Autodesk Inventor part; units mm, degrees
ref_plane "YZ Plane" through (0, 0, 0) normal (1, 0, 0) x (0, 1, 0)
ref_plane "XZ Plane" through (0, 0, 0) normal (0, 1, 0) x (-1, 0, 0)
ref_plane "XY Plane" through (0, 0, 0) normal (0, 0, 1) x (1, 0, 0)
sketch "スケッチ1" plane through (0, 0, 0) normal (0, 0, 1) x (1, 0, 0)
  line L0 (-50, 0) -> (50, 0) construction
  circle A0 centre (-50, 0) radius 4.05
  circle A1 centre (50, 0) radius 4.05
  line L1 (-50, 8.5) -> (43, 8.5)
  line L2 (-50, -8.5) -> (43, -8.5)
  arc A2 (-50, 8.5) -> (-50, -8.5) centre (-50, 0) ccw
  line L3 (43, -8.5) -> (50.119, -8.3992)
  line L4 (43, 8.5) -> (50.119, 8.3992)
  arc A3 (50.119, -8.3992) -> (50.119, 8.3992) centre (50, 0) ccw
  line L5 (-29, -7.5) -> (0, -7.5) construction
  line L6 (0, -7.5) -> (0, -2.5) construction
  line L7 (0, -2.5) -> (-29, -2.5) construction
  line L8 (-29, -2.5) -> (-29, -7.5) construction
  line L9 (-29, -5) -> (0, -5) construction
  circle A4 centre (-26.5, -5) radius 1.55
  line L10 (-14.5, -5) -> (-14.5, -2.5) construction
  line L11 (52.3191, 13) -> (22.3191, 13)
  line L12 (22.3191, 13) -> (12.3191, 8.5)
  line L13 (52.3191, 13) -> (57.3191, 4.122)
  circle A5 centre (-2.5, -5) radius 1.55
  point P0 (0, 0)
  point P1 (0, 0)
  point P2 (54.8534, 8.5)
  dimension "d0" = 100
  dimension "d1" = 8.1
  dimension "d2" = 8.5
  dimension "d8" = 8.1
  dimension "d9" = 7
  dimension "d10" = 8.4
  dimension "d12" = 5
  dimension "d13" = 29
  dimension "d15" = 2.5
  dimension "d17" = 13
  dimension "d19" = 10
  dimension "d20" = 30
  dimension "d25" = 50
  dimension "d26" = 5
  dimension "d45" = 1
  dimension "d46" = 3.1
extrude "押し出し1" add sketch "スケッチ1" along normal blind 2 contours L1 L4 A3 L3 L2 A2
fillet "フィレット1" radius 2 1 edges at (43, 8.5, 1)
sketch "スケッチ2" plane through (0, 0, 0) normal (0, 0, -1) x (-1, 0, 0)
  circle A0 centre (-16.6795, 17.7128) radius 11.35 construction
  circle A1 centre (-16.6795, 17.7128) radius 11.55
  line L0 (-16.6795, 6.1628) -> (58.7547, 6.1628)
  line L1 (-16.6795, 17.7128) -> (-34, 27.7128) construction
  circle A2 centre (-50, 0) radius 4.05
  line L2 (-50, 0) -> (-34, 27.7128) construction
  line L3 (50, -8.5) -> (-43, -8.5)
  line L4 (-2.1795, 10.6628) -> (35.8205, 10.6628)
  line L5 (35.8205, 10.6628) -> (45.8205, 6.1628)
  line L6 (-2.1795, 10.6628) -> (-12.1795, 6.1628)
  circle A3 centre (50, 0) radius 4.05
  line L7 (58.7547, 6.1628) -> (-13.2236, 28.7337)
  arc A4 (50, -8.5) -> (50, 8.5) centre (50, 0) ccw
  point P0 (0, 0)
  dimension "d29" = 22.7
  dimension "d30" = 0.2
  dimension "d31" = 60
  dimension "d32" = 90
  dimension "d33" = 20
  dimension "d34" = 38
  dimension "d35" = 10
  dimension "d36" = 10
  dimension "d37" = 4.5
  dimension "d38" = 32
  dimension "d40" = 4.5
extrude "押し出し2" cut sketch "スケッチ2" against normal through all contours A1 | A1 L7 A4 L0 L5 L4 L6 | L7 L0 A4
fillet "フィレット2" radius 2 2 edges at (12.1795, 6.1628, 1) (-45.8205, 6.1628, 1)
equation "\"d8\" = d1"
equation "\"d19\" = d18"
equation "\"d36\" = d35"
properties part number "リンク_メインフレーム_6_1" material "GFRP"
Geometry: final body of the model. Coordinates: model frame, mm. A direction names the side the tool comes from. Give positions to 0.01 mm unless a question says otherwise; leave off trailing zeros. Write each loop counter-clockwise with the first axis right and the second up, starting at its lowest first coordinate (ties: lowest second). Pieces come first, ordered by that corner, then holes.
1. Section query C-C, the plane x = -2.5. Return loops of the section in (y, z).
2. Pin query (flat end, axial travel): P1, Ø0.6, axis at x = 15.5, z = 1.5, coming from the +Y side; P2, Ø1, axis at y = -5.5, z = 1, coming from the +X side. Return the tip coordinate at first contact, or that it passes through.
3. Section query D-D, the plane x = 15.5. Return loops of the section in (y, z).
4. Draft query along X for faces 1 (the cylindrical face through (58.4, 0.18, 0.99)), 2 (the flat face through (15, 6.163, 1)), 3 (the flat face through (-1, 0, 2)), 4 (the cylindrical face through (-57.84, -3.28, 0.99)). Return one class per face: released by +X, released by -X, zero draft, split by the parting line, or undercut.
5. Line query: probe 1 along Y at (x, z) = (-50, 0.85); probe 2 along Y at (x, z) = (-2.5, 1); probe 3 along X at (y, z) = (3.25, 0.5). Output: solid intervals per line, ascending.
6. Section query A-A, the plane y = 0. Return loops of the section in (x, z).
7. Reachability of faces 5 (the flat face through (9.353, 7.435, 0.986)), 6 (the cylindrical face through (46.786, 2.464, 0.986)), 7 (the flat face through (-51, 6.163, 1)) from +Z, -Z, +X, -X, +Y, -Y: full face, straight path, thin tool, end or side. Return the list, or none.
8. Section query B-B, the plane z = 1.4. Count the separate pieces of the cut face and the enclosed holes in it, then the cut area to 3 significant figures.
Computed:
1. outline: (-8.5, 0) - (-6.55, 0) - (-6.55, 2) - (-8.5, 2) - close; (-3.45, 0) - (8.5, 0) - (8.5, 2) - (-3.45, 2) - close
2. P1: stops at y = 6.16
2. P2: stops at x = 56.75
3. outline: (-8.5, 0) - (6.16, 0) - (6.16, 2) - (-8.5, 2) - close
4. face 1: released by +X
4. face 2: undercut
4. face 3: zero draft
4. face 4: released by -X
5. probe 1: y = -8.5 to -4.05, 4.05 to 6.16
5. probe 2: y = -8.5 to -6.55, -3.45 to 8.5
5. probe 3: x = -57.85 to -52.42, -47.58 to 47.58, 52.42 to 57.75
6. outline: (-58.5, 0) - (-54.05, 0) - (-54.05, 2) - (-58.5, 2) - close; (-45.95, 0) - (45.95, 0) - (45.95, 2) - (-45.95, 2) - close; (54.05, 0) - (58.4, 0) - (58.4, 2) - (54.05, 2) - close
7. face 5: +Z, -Z, +Y
7. face 6: +Z, -Z
7. face 7: +Z, -Z, -X, +Y
8. separate pieces: 1
8. enclosed holes: 4
8. area: 1,750 mm2
